Input: part model. Units: mm. Frame: model coordinates. Coordinates: 2 decimals unless noted, no trailing zeros. Order: outer loops, then holes, each group sorted by start corner. A loop starts at its lowest first (then second) coordinate and runs counter-clockwise, first axis right, second up. Notation, with made-up numbers: (5.25, 44) -> (48.25, 44) arc R18 ccw to (48.25, 59) -> close; hole circle Ø1 at (26, -35). An arc over 180 degrees is marked (long way). Answer as CSV lines item,"result".
from build123d import *

# Parameters (mm, degrees)
SKETCH_1_R      = 1.6
SKETCH_1_R_2    = 2.6
EXTRUDE_1_DEPTH = 4


with BuildPart() as part:
    # 草图1 → 凸台-拉伸1 (new body)
    with BuildSketch(Plane(origin=(0, 0, 0), x_dir=(0, 0, -1), z_dir=(1, 0, 0))):
        with BuildLine():
            Line((8.104883027, 1.878840053), (27.795402052, 14.878840053))
            Line((27.795402052, 14.878840053), (27.795402052, 27.878840053))
            Line((27.795402052, 27.878840053), (-34.204597948, 27.878840053))
            ThreePointArc((-34.204597948, 27.878840053), (-41.551421317, 23.044939607), (-40.019791495, 14.384886649))
            Line((-40.019791495, 14.384886649), (-31.164108907, 5.011398298))
            ThreePointArc((-31.164108907, 5.011398298), (-27.852741415, 2.695310842), (-23.895116973, 1.878840053))
            Line((-23.895116973, 1.878840053), (8.104883027, 1.878840053))
        make_face()
        with Locations((23.795402052, 23.878840053)):
            Circle(SKETCH_1_R, mode=Mode.SUBTRACT)
        with Locations((-10.204597948, 23.878840053)):
            Circle(SKETCH_1_R, mode=Mode.SUBTRACT)
        with Locations((8.595402052, 12.878840053)):
            Circle(SKETCH_1_R, mode=Mode.SUBTRACT)
        with Locations((-11.104597948, 7.878840053)):
            Circle(SKETCH_1_R, mode=Mode.SUBTRACT)
        with Locations((-34.204597948, 19.878840053)):
            Circle(SKETCH_1_R_2, mode=Mode.SUBTRACT)
    extrude(amount=EXTRUDE_1_DEPTH)


solid = part.part
1. Cut plane B-B (y = 21.5). Return the cut outline in (x, z), plus the area to 3 significant figures.
Findings:
outline,"(0, -27.8) -> (4, -27.8) -> (4, 32.17) -> (0, 32.17) -> close; (0, 36.24) -> (4, 36.24) -> (4, 42.04) -> (0, 42.04) -> close"
area,"263 mm2"
2. Cut plane A-A (x = 1.2). Return the cut outline in (y, z).
Findings:
outline,"(1.88, -8.1) -> (14.88, -27.8) -> (27.88, -27.8) -> (27.88, 34.2) arc R8 ccw to (14.38, 40.02) -> (5.01, 31.16) arc R10 ccw to (1.88, 23.9) -> close; hole circle Ø3.2 at (7.88, 11.1); hole circle Ø3.2 at (12.88, -8.6); hole circle Ø5.2 at (19.88, 34.2); hole circle Ø3.2 at (23.88, -23.8); hole circle Ø3.2 at (23.88, 10.2)"
3. Ray query, line 1 along Z through (x, y) = (0.4, 25); line 2 along Z through (x, y) = (0.45, 23.5); line 3 along Y through (x, z) = (0.7, -8). Return the intervals inside material, ascending.
Findings:
line 1,"z = -27.8 to -24.94, -22.65 to 9.06, 11.35 to 40.35"
line 2,"z = -27.8 to -25.35, -22.24 to 8.65, 11.76 to 41.34"
line 3,"y = 1.88 to 11.39, 14.36 to 27.88"
4. Cut plane D-D (y = 15.5). Return the cut outline in (x, z).
Findings:
outline,"(0, -27.8) -> (4, -27.8) -> (4, 40.9) -> (0, 40.9) -> close"
5. Cut plane C-C (z = 30). Return the cut outline in (x, y), plus the area to 3 significant figures.
Findings:
outline,"(0, 3.96) -> (4, 3.96) -> (4, 27.88) -> (0, 27.88) -> close"
area,"95.7 mm2"
6. Contact query for a flat-ended pin moving along its axis: pin 1 (1.5 mm diameter, centred on x = 1.5, y = 12, fed in from +Z). Output: stop coordinate, or through.
Findings:
pin 1,"stops at z = 38.48"
7. Mould query, pull axis Y, two halves, no side actions, for faces 1 (the face through (1.972, 23.266, -25.273)), 2 (the face through (1.97, 9.76, 35.65)), 3 (the face through (1.972, 7.949, 12.703)), 4 (the face through (4, 15, 8)). Classes: released by +Y, released by -Y, zero draft, split by the parting line, or undercut.
Findings:
face 1,"undercut"
face 2,"released by -Y"
face 3,"undercut"
face 4,"zero draft"
